from build123d import *

# Parameters (mm, degrees)
SKETCH_1_W          = 30
SKETCH_1_H          = 15
EXTRUDE_1_DEPTH     = 5
CUT_EXTRUDE_1_DEPTH = 9.45
CUT_EXTRUDE_2_DEPTH = 9.45
FILLET_1_R          = 0.2


with BuildPart() as part:
    # 草图1 → 凸台-拉伸1 (new body)
    with BuildSketch(Plane(origin=(0, 0, 0), x_dir=(1, 0, 0), z_dir=(0, 1, 0))):
        with Locations((0, 7.5)):
            Rectangle(SKETCH_1_W, SKETCH_1_H)
    extrude(amount=EXTRUDE_1_DEPTH)

    # 草图2 → 切除-拉伸1 (cut)
    with BuildSketch(Plane.XY):
        with BuildLine():
            Line((-1.5, 5), (-1.5, 4.322875656))
            ThreePointArc((-1.5, 4.322875656), (-1.780042303, 3.911838473), (-1.95, 3.444409721))
            Line((-1.95, 3.444409721), (-1.95, 2.2))
            Line((-1.95, 2.2), (1.95, 2.2))
            Line((1.95, 2.2), (1.95, 3.444409721))
            ThreePointArc((1.95, 3.444409721), (1.780042303, 3.911838473), (1.5, 4.322875656))
            Line((1.5, 4.322875656), (1.5, 5))
            Line((1.5, 5), (-1.5, 5))
        make_face()
    extrude(amount=-CUT_EXTRUDE_1_DEPTH, mode=Mode.SUBTRACT)

    # 草图3 → 切除-拉伸2 (cut)
    with BuildSketch(Plane(origin=(0, 0, -15), x_dir=(-1, 0, 0), z_dir=(0, 0, -1))):
        with BuildLine():
            Line((-9, 0), (-9, 0.677124344))
            ThreePointArc((-9, 0.677124344), (-9.280042303, 1.088161527), (-9.45, 1.555590279))
            Line((-9.45, 1.555590279), (-9.45, 2.8))
            Line((-9.45, 2.8), (-5.55, 2.8))
            Line((-5.55, 2.8), (-5.55, 1.555590279))
            ThreePointArc((-5.55, 1.555590279), (-5.719957697, 1.088161527), (-6, 0.677124344))
            Line((-6, 0.677124344), (-6, 0))
            Line((-6, 0), (-9, 0))
        make_face()
        with BuildLine():
            Line((9, 0), (6, 0))
            Line((6, 0), (6, 0.677124344))
            ThreePointArc((6, 0.677124344), (5.719957697, 1.088161527), (5.55, 1.555590279))
            Line((5.55, 1.555590279), (5.55, 2.8))
            Line((5.55, 2.8), (9.45, 2.8))
            Line((9.45, 2.8), (9.45, 1.555590279))
            ThreePointArc((9.45, 1.555590279), (9.280042303, 1.088161527), (9, 0.677124344))
            Line((9, 0.677124344), (9, 0))
        make_face()
    extrude(amount=-CUT_EXTRUDE_2_DEPTH, mode=Mode.SUBTRACT)

    # 圆角1
    fillet_1_edges = [part.edges().sort_by_distance(p)[0] for p in [
        (15, 5, -7.5),
        (0, 5, -15),
        (8.25, 5, 0),
        (0, 5, -9.45),
        (-1.5, 5, -4.725),
        (1.5, 5, -4.725),
        (0, 0, -15),
        (-15, 5, -7.5),
        (7.5, 0, -5.55),
        (6, 0, -10.275),
        (9, 0, -10.275),
        (12, 0, -15),
        (15, 0, -7.5),
        (0, 0, 0),
        (-15, 0, -7.5),
        (-12, 0, -15),
        (-7.5, 0, -5.55),
        (-9, 0, -10.275),
        (-6, 0, -10.275),
        (-8.25, 5, 0),
        (-15, 2.5, -15),
        (15, 2.5, -15),
        (15, 2.5, 0),
        (-15, 2.5, 0),
    ]]
    fillet(fillet_1_edges, radius=FILLET_1_R)


solid = part.part
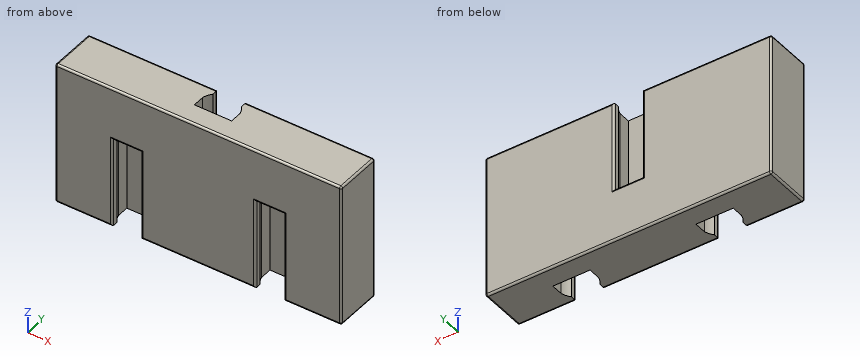
Design review of the part built by this model. Coordinates are the model's own, in mm. Round coordinates to 2 decimals unless told otherwise and drop trailing zeros. Write each loop counter-clockwise with the first axis right and the second up, starting at its lowest first coordinate (ties: lowest second). Pieces come first, ordered by that corner, then holes. Notation, with made-up numbers: (30.5, 23) - (69.5, 23) arc R31 ccw to (69.5, 57) - close; hole circle Ø10 at (66, 37.5). An arc over 180 degrees is marked (long way). Return JSON: item names as keys, results as strings. Group by question number.
Item 1: We need section A-A on z = -12.75. Write out the cut boundary in (x, y), and give its area (3 significant figures).
Item 2: We need section B-B on x = 8.25. Write out the cut boundary in (y, z).
Item 3: We need section C-C on y = 3.15. Write out the cut boundary in (x, z).
Item 4: We need section D-D on z = -4. Write out the cut boundary in (x, y), and give its area (3 significant figures).
Item 5: Insertion check: P1, Ø2, axis at x = -0.5, y = 3.5, coming from the +Z side; P2, Ø1.3, axis at x = -8, y = 2, coming from the -Z side. Each pin has a flat end and moves straight along its axis. Give the tip position at first contact, or say it passes through.
Item 6: For probe 1 along X at (y, z) = (1.75, -9.25); probe 2 along X at (y, z) = (2.25, -6.5); probe 3 along X at (y, z) = (1.15, -6.25), list the stretches that pass through material, from the lowest coordinate up. Write a range as [from, to].
Model answer:
{
 "1": {"outline": "(-15, 0.2) arc R0.2 ccw to (-14.8, 0) - (-9.2, 0) arc R0.2 ccw to (-9, 0.2) - (-9, 0.68) arc R2 cw to (-9.45, 1.56) - (-9.45, 2.8) - (-5.55, 2.8) - (-5.55, 1.56) arc R2 cw to (-6, 0.68) - (-6, 0.2) arc R0.2 ccw to (-5.8, 0) - (5.8, 0) arc R0.2 ccw to (6, 0.2) - (6, 0.68) arc R2 cw to (5.55, 1.56) - (5.55, 2.8) - (9.45, 2.8) - (9.45, 1.56) arc R2 cw to (9, 0.68) - (9, 0.2) arc R0.2 ccw to (9.2, 0) - (14.8, 0) arc R0.2 ccw to (15, 0.2) - (15, 4.8) arc R0.2 ccw to (14.8, 5) - (-14.8, 5) arc R0.2 ccw to (-15, 4.8) - close", "area": "130 mm²"},
 "2": {"outline": "(0, -5.35) arc R0.2 ccw to (0.2, -5.55) - (2.8, -5.55) - (2.8, -15) - (4.8, -15) arc R0.2 ccw to (5, -14.8) - (5, -0.2) arc R0.2 ccw to (4.8, 0) - (0.2, 0) arc R0.2 ccw to (0, -0.2) - close"},
 "3": {"outline": "(-15, -14.8) arc R0.2 ccw to (-14.8, -15) - (14.8, -15) arc R0.2 ccw to (15, -14.8) - (15, -0.2) arc R0.2 ccw to (14.8, 0) - (1.95, 0) - (1.95, -9.45) - (-1.95, -9.45) - (-1.95, 0) - (-14.8, 0) arc R0.2 ccw to (-15, -0.2) - close"},
 "4": {"outline": "(-15, 0.2) arc R0.2 ccw to (-14.8, 0) - (14.8, 0) arc R0.2 ccw to (15, 0.2) - (15, 4.8) arc R0.2 ccw to (14.8, 5) - (1.7, 5) arc R0.2 ccw to (1.5, 4.8) - (1.5, 4.32) arc R2 cw to (1.95, 3.44) - (1.95, 2.2) - (-1.95, 2.2) - (-1.95, 3.44) arc R2 cw to (-1.5, 4.32) - (-1.5, 4.8) arc R0.2 ccw to (-1.7, 5) - (-14.8, 5) arc R0.2 ccw to (-15, 4.8) - close", "area": "140 mm²"},
 "5": {"P1": "stops at z = -9.45", "P2": "stops at z = -5.55"},
 "6": {"probe 1": "x = [-15, -9.45], [-5.55, 5.55], [9.45, 15]", "probe 2": "x = [-15, -9.45], [-5.55, -1.95], [1.95, 5.55], [9.45, 15]", "probe 3": "x = [-15, -9.31], [-5.69, 5.69], [9.31, 15]"}
}
